```python
from build123d import *

# Parameters (mm, degrees)
BASE_EXTRUSION_DEPTH = 40
CHANFREIN1_SIZE      = 1


with BuildPart() as part:
    # Esquisse1 → Base-Extrusion (new body)
    with BuildSketch(Plane.XY):
        with BuildLine():
            Line((15.5, 12.239791665), (15.5, 9.5))
            Line((15.5, 9.5), (11.608186766, 9.5))
            ThreePointArc((11.608186766, 9.5), (0, 15), (-11.608186766, 9.5))
            Line((-11.608186766, 9.5), (-15.5, 9.5))
            Line((-15.5, 9.5), (-15.5, 12.239791665))
            ThreePointArc((-15.5, 12.239791665), (0, 19.75), (15.5, 12.239791665))
        make_face()
    extrude(amount=BASE_EXTRUSION_DEPTH)

    # Chanfrein1
    chanfrein1_edges = [part.edges().sort_by_distance(p)[0] for p in [
        (15.5, 10.869895832, 0),
        (15.5, 10.869895832, 40),
        (13.554093383, 9.5, 0),
        (13.554093383, 9.5, 40),
        (0, 15, 0),
        (0, 15, 40),
        (-13.554093383, 9.5, 0),
        (-13.554093383, 9.5, 40),
        (-15.5, 10.869895832, 0),
        (-15.5, 10.869895832, 40),
        (0, 19.75, 0),
        (0, 19.75, 40),
    ]]
    chamfer(chanfrein1_edges, length=CHANFREIN1_SIZE)


solid = part.part
```
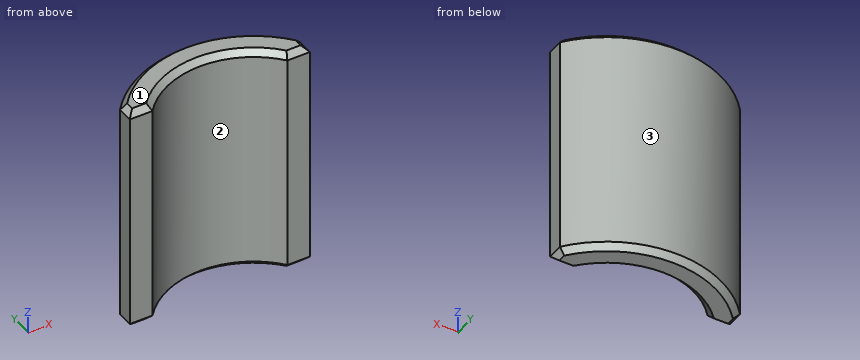
Model file for the job. Use its own axes, mm. Face numbers are marked on the shaded views. Give positions to 0.01 mm unless a question says otherwise; leave off trailing zeros. Loops run counter-clockwise (first coordinate to the right, second up) from the corner with the lowest first, then second, coordinate; pieces in that order, holes last. Notation, with made-up numbers: (72.5, 40.5) -> (108.5, 40.5) arc R8 cw to (108.5, 44.5) -> close; hole circle Ø2 at (52.25, 6). An arc over 180 degrees is marked (long way). Use CSV: the item, a comma, the result in double quotes. Start each with the question number.
1) Wall check: line 1 (X direction, y = 11.75, z = 17); line 2 (X direction, y = 12.25, z = 27.5); line 3 (Y direction, x = -13, z = 34). Give the ranges that are in metal, low to high.
2) Slice it at A-A on z = 6.5. Give the cut face in (x, y), plus the area to 3 significant figures.
3) Flat gauge pins, fed straight in: pin 1 Ø6 at (x, z) = (-6, 30.5) entering from -Y; pin 2 Ø1 at (y, z) = (13, 34) entering from +X; pin 3 Ø4 at (y, z) = (16.5, 10) entering from +X. Where does each tip first touch, or does it go through?
4) Mould opens along X. For the marked faces 1, 2 and 3 say: released by +X, released by -X, zero draft, split by the parting line, or undercut.
Computed values:
1,line 1,"x = -15.5 to -9.32, 9.32 to 15.5"
1,line 2,"x = -15.49 to -8.66, 8.66 to 15.49"
1,line 3,"y = 9.5 to 14.87"
2,outline,"(-15.5, 9.5) -> (-11.61, 9.5) arc R15 cw to (11.61, 9.5) -> (15.5, 9.5) -> (15.5, 12.24) arc R19.75 ccw to (-15.5, 12.24) -> close"
2,area,"158 mm^2"
3,pin 1,"stops at y = 12"
3,pin 2,"stops at x = 15.29"
3,pin 3,"stops at x = 13.41"
4,face 1,"zero draft"
4,face 2,"undercut"
4,face 3,"split by the parting line"
